Design review of the part built by this model. Coordinates are the model's own, in mm. A direction names the side the tool comes from. Coordinates: 2 decimals unless noted, no trailing zeros. Loops run counter-clockwise (first coordinate to the right, second up) from the corner with the lowest first, then second, coordinate; pieces in that order, holes last. Notation, with made-up numbers: (50.5, 8.5) - (63.5, 8.5) arc R18 ccw to (63.5, 30.5) - close; hole circle Ø10 at (11, 88.25). An arc over 180 degrees is marked (long way). Answer in a Markdown table with one row per item. Add a question column.
(1) To check wall thickness, follow L1, parallel to Y at x = -8, z = 1.9; L2, parallel to Y at x = 0, z = 1.3; L3, parallel to Y at x = -1, z = -3.5. State the ranges of each line that lie inside material, in increasing order. Write a range as [from, to].
(2) We need section A-A, the plane x = 8. Write out the cut boundary in (y, z), plus the area to 3 significant figures.
(3) For faces 5 (the face through (-8, 15, -2)), 6 (the face through (8, -11, -2)), 7 (the face through (11.9, 2.2, -1.7)), 8 (the face through (1.97, 32.97, -12.98)), list the 3-axis set-ups (+Z, -Z, +X, -X, +Y, -Y) from which the entire face can be reached by the end or side of a thin tool; tool diameter is ignored.
(4) The part is to be moulded in two halves that separate along X. For faces 1 (the face through (9, 35, -2)), 2 (the face through (-8.221, -16.314, 1.479)), 3 (the face through (-7, 35, -9)), 4 (the face through (-0.221, 23.686, 1.479)), say which applies: released by +X, released by -X, zero draft, split by the parting line, or undercut.
(5) We need section B-B, the plane z = 1.5. Write out the cut boundary in (x, y).
(6) We need section C-C, the plane y = 0. Write out the cut boundary in (x, z).
(7) We need section D-D, the plane y = -18. Write out the cut boundary in (x, z).
(8) Clearance check with flat-ended pins moving along their axes: pin 1 (4.5 mm diameter, centred on x = -8, y = -18, fed in from -Z); pin 2 (3 mm diameter, centred on x = 0, y = 22, fed in from +Z); pin 3 (6 mm diameter, centred on x = 0, z = -9.5, fed in from -Y); pin 4 (4 mm diameter, centred on y = 35.5, z = -8.5, fed in from +X). State where each tip first meets the part, or that it passes through.
from build123d import *

# Parameters (mm, degrees)
SKETCH_1_R          = 1.7
SKETCH_1_R_2        = 2.7
EXTRUDE_1_DEPTH     = 3
SKETCH_3_W          = 14
SKETCH_3_H          = 8
EXTRUDE_2_DEPTH     = 17
CUT_EXTRUDE_1_DEPTH = 4
CUT_EXTRUDE_2_REACH = 64.274
SKETCH_6_R          = 2.7
FILLET_1_R          = 3
CHAMFER_1_SIZE      = 4
SKETCH_7_W          = 6.9
SKETCH_7_H          = 26
EXTRUDE_3_DEPTH     = 3.4
EXTRUDE_4_DEPTH     = 26


with BuildPart() as part:
    # 草图1 → 凸台-拉伸1 (new body)
    with BuildSketch(Plane.XY):
        Polygon((-15, 27), (-15, -23), (15, -23), (15, 27), (15, 39), (-15, 39), align=None)
        with Locations((-8, -18)):
            Circle(SKETCH_1_R, mode=Mode.SUBTRACT)
        with Locations((0, -18)):
            Circle(SKETCH_1_R, mode=Mode.SUBTRACT)
        with Locations((8, -18)):
            Circle(SKETCH_1_R, mode=Mode.SUBTRACT)
        with Locations((-8, 22)):
            Circle(SKETCH_1_R, mode=Mode.SUBTRACT)
        Circle(SKETCH_1_R_2, mode=Mode.SUBTRACT)
        with Locations((0, 22)):
            Circle(SKETCH_1_R, mode=Mode.SUBTRACT)
        with Locations((8, 22)):
            Circle(SKETCH_1_R, mode=Mode.SUBTRACT)
    extrude(amount=EXTRUDE_1_DEPTH)

    # 草图3 → 凸台-拉伸2 (add)
    with BuildSketch(Plane(origin=(0, 0, 0), x_dir=(-1, 0, 0), z_dir=(0, 0, -1))):
        with Locations((0, 35)):
            Rectangle(SKETCH_3_W, SKETCH_3_H)
    extrude(amount=EXTRUDE_2_DEPTH)

    # 草图5 → 切除-拉伸1 (cut)
    with BuildSketch(Plane.XZ.offset(-31)):
        Polygon((4, -11.809401077), (4, -7.190598923), (0, -4.881197846), (-4, -7.190598923), (-4, -11.809401077), (0, -14.118802154), align=None)
    extrude(amount=-CUT_EXTRUDE_1_DEPTH, mode=Mode.SUBTRACT)

    # 草图6 → 切除-拉伸2 (cut, up to next)
    with BuildSketch(Plane.XZ.offset(-35), mode=Mode.PRIVATE) as cut_extrude_2_sk1:
        with Locations(Location((0, -9.5, 0), (0, 0, 270))):
            Circle(SKETCH_6_R)
    cut_extrude_2_tool1 = extrude(cut_extrude_2_sk1.sketch, amount=-CUT_EXTRUDE_2_REACH, mode=Mode.PRIVATE) & part.part
    add(cut_extrude_2_tool1.solids().sort_by_distance((0, 35, -9.5))[0], mode=Mode.SUBTRACT)

    # 圆角1
    fillet_1_edges = [part.edges().sort_by_distance(p)[0] for p in [
        (-7, 35, -17),
        (7, 35, -17),
    ]]
    fillet(fillet_1_edges, radius=FILLET_1_R)

    # 倒角1
    chamfer_1_edges = [part.edges().sort_by_distance(p)[0] for p in [
        (-7, 35, 0),
        (7, 35, 0),
    ]]
    chamfer(chamfer_1_edges, length=CHAMFER_1_SIZE)

    # 草图7 → 凸台-拉伸3 (add)
    with BuildSketch(Plane(origin=(0, 0, 0), x_dir=(-1, 0, 0), z_dir=(0, 0, -1))):
        with Locations((-8, 2)):
            Rectangle(SKETCH_7_W, SKETCH_7_H)
        with Locations((8, 2)):
            Rectangle(SKETCH_7_W, SKETCH_7_H)
    extrude(amount=EXTRUDE_3_DEPTH)

    # 草图8 → 凸台-拉伸4 (add)
    with BuildSketch(Plane(origin=(0, 15, 0), x_dir=(1, 0, 0), z_dir=(0, 1, 0))):
        Polygon((11.45, 0), (11.45, 3.4), (12.35, 3.4), align=None)
        Polygon((3.65, 3.4), (4.55, 0), (4.55, 3.4), align=None)
        Polygon((-12.35, 3.4), (-11.45, 0), (-11.45, 3.4), align=None)
        Polygon((-4.55, 0), (-4.55, 3.4), (-3.65, 3.4), align=None)
    extrude(amount=-EXTRUDE_4_DEPTH)


solid = part.part
Responses:
| question | item | result |
|---|---|---|
| 1 | L1 | y = [-23, -19.7], [-16.3, 20.3], [23.7, 39] |
| 1 | L2 | y = [-23, -19.7], [-16.3, -2.7], [2.7, 20.3], [23.7, 39] |
| 1 | L3 | y = [31, 39] |
| 2 | outline | (-23, 0) - (-19.7, 0) - (-19.7, 3) - (-23, 3) - close; (-16.3, 0) - (-11, 0) - (-11, -3.4) - (15, -3.4) - (15, 0) - (20.3, 0) - (20.3, 3) - (-16.3, 3) - close; (23.7, 0) - (31, 0) - (31, -3) - (39, -3) - (39, 3) - (23.7, 3) - close |
| 2 | area | 278 mm2 |
| 3 | face 5 | -Z, +X, -X |
| 3 | face 6 | -Z, +X, -X, -Y |
| 3 | face 7 | +X, +Y, -Y |
| 3 | face 8 | -Y |
| 4 | face 1 | released by +X |
| 4 | face 2 | undercut |
| 4 | face 3 | released by -X |
| 4 | face 4 | undercut |
| 5 | outline | (-15, -23) - (15, -23) - (15, 39) - (-15, 39) - close; hole circle Ø3.4 at (-8, -18); hole circle Ø3.4 at (-8, 22); hole circle Ø5.4 at (0, 0); hole circle Ø3.4 at (0, -18); hole circle Ø3.4 at (0, 22); hole circle Ø3.4 at (8, -18); hole circle Ø3.4 at (8, 22) |
| 6 | outline | (-15, 0) - (-11.45, 0) - (-12.35, -3.4) - (-3.65, -3.4) - (-4.55, 0) - (-2.7, 0) - (-2.7, 3) - (-15, 3) - close; (2.7, 0) - (4.55, 0) - (3.65, -3.4) - (12.35, -3.4) - (11.45, 0) - (15, 0) - (15, 3) - (2.7, 3) - close |
| 7 | outline | (-15, 0) - (-9.7, 0) - (-9.7, 3) - (-15, 3) - close; (-6.3, 0) - (-1.7, 0) - (-1.7, 3) - (-6.3, 3) - close; (1.7, 0) - (6.3, 0) - (6.3, 3) - (1.7, 3) - close; (9.7, 0) - (15, 0) - (15, 3) - (9.7, 3) - close |
| 8 | pin 1 | stops at z = 0 |
| 8 | pin 2 | passes through |
| 8 | pin 3 | stops at y = 35 |
| 8 | pin 4 | stops at x = 7 |
